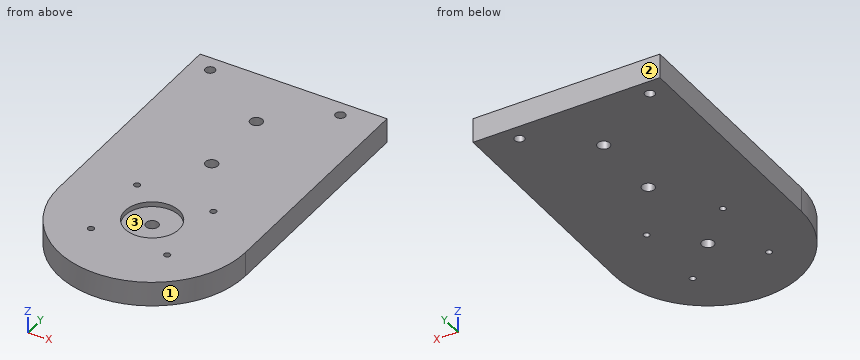
```python
from build123d import *

# Parameters (mm, degrees)
CROQUIS1_R              = 2.5
CROQUIS1_R_2            = 1.25
SALIENTE_EXTRUIR1_DEPTH = 10
CROQUIS3_R              = 11
CORTAR_EXTRUIR1_DEPTH   = 2
CROQUIS4_R              = 2
CORTAR_EXTRUIR2_DEPTH   = 103.805641869


with BuildPart() as part:
    # Croquis1 → Saliente-Extruir1 (new body)
    with BuildSketch(Plane.XY):
        with BuildLine():
            Line((-38, 0), (-38, 95))
            Line((-38, 95), (38, 95))
            Line((38, 95), (38, 0))
            ThreePointArc((38, 0), (0, -38), (-38, 0))
        make_face()
        with Locations((0, 40)):
            Circle(CROQUIS1_R, mode=Mode.SUBTRACT)
        Circle(CROQUIS1_R, mode=Mode.SUBTRACT)
        with Locations((0, 70)):
            Circle(CROQUIS1_R, mode=Mode.SUBTRACT)
        with Locations((-15.5, 15.5)):
            Circle(CROQUIS1_R_2, mode=Mode.SUBTRACT)
        with Locations((15.5, 15.5)):
            Circle(CROQUIS1_R_2, mode=Mode.SUBTRACT)
        with Locations((15.5, -15.5)):
            Circle(CROQUIS1_R_2, mode=Mode.SUBTRACT)
        with Locations((-15.5, -15.5)):
            Circle(CROQUIS1_R_2, mode=Mode.SUBTRACT)
    extrude(amount=SALIENTE_EXTRUIR1_DEPTH)

    # Croquis3 → Cortar-Extruir1 (cut)
    with BuildSketch(Plane.XY.offset(10)):
        Circle(CROQUIS3_R)
    extrude(amount=-CORTAR_EXTRUIR1_DEPTH, mode=Mode.SUBTRACT)

    # Croquis4 → Cortar-Extruir2 (cut, through all)
    with BuildSketch(Plane.XY.offset(10)):
        with Locations((-30, 88.5)):
            Circle(CROQUIS4_R)
        with Locations((23, 88.5)):
            Circle(CROQUIS4_R)
    extrude(amount=-CORTAR_EXTRUIR2_DEPTH, mode=Mode.SUBTRACT)


solid = part.part
```
Source: CAD feature listing. Evaluate the final solid. Frame: model axes, mm. Face numbers are marked on the shaded views. Coordinates: 2 decimals unless noted, no trailing zeros. Loops run counter-clockwise (first coordinate to the right, second up) from the corner with the lowest first, then second, coordinate; pieces in that order, holes last. Notation, with made-up numbers: M -25.75,77 L 20.25,77 A25 cw 20.25,96 Z; hole C 33.25,-14 d8. An arc over 180 degrees is marked long. Use a Markdown table: item, result. Add a question column.
Q1. Draft query along Y for the marked faces 1, 2 and 3. Return one class per face: pulls with the +Y half, pulls with the -Y half, needs draft (parallel to the pull), parting line crosses it, or undercut.
Q2. Section query C-C, the plane y = 40. Return loops of the section in (x, z), and give its area (3 significant figures).
Q3. Section query B-B, the plane x = -30. Return loops of the section in (y, z).
Q4. Material intervals for L1, parallel to Y at x = 0, z = 9.65; L2, parallel to Y at x = 0, z = 5.5; L3, parallel to Y at x = 15.5, z = 6, sorted ascending.
Q5. First-contact query: pin 1 (6.5 mm diameter, centred on x = -4, y = 5, fed in from +Z). Flat tip, straight axial feed; report the tip coordinate or a pass-through.
Q6. Section query D-D, the plane z = 6.5. State how many separate pieces and enclosed holes the cut face has, and give its area (3 significant figures).
Q7. Section query A-A, the plane y = 15.5. Return loops of the section in (x, z), and give its area (3 significant figures).
Result:
| question | item | result |
|---|---|---|
| 1 | face 1 | pulls with the -Y half |
| 1 | face 2 | pulls with the +Y half |
| 1 | face 3 | undercut |
| 2 | outline | M -38,0 L -2.5,0 L -2.5,10 L -38,10 Z; M 2.5,0 L 38,0 L 38,10 L 2.5,10 Z |
| 2 | area | 710 mm2 |
| 3 | outline | M -23.32,0 L 86.5,0 L 86.5,10 L -23.32,10 Z; M 90.5,0 L 95,0 L 95,10 L 90.5,10 Z |
| 4 | L1 | y = -38 to -11, 11 to 37.5, 42.5 to 67.5, 72.5 to 95 |
| 4 | L2 | y = -38 to -2.5, 2.5 to 37.5, 42.5 to 67.5, 72.5 to 95 |
| 4 | L3 | y = -34.7 to -16.75, -14.25 to 14.25, 16.75 to 95 |
| 5 | pin 1 | stops at z = 8 |
| 6 | separate pieces | 1 |
| 6 | enclosed holes | 9 |
| 6 | area | 9,380 mm2 |
| 7 | outline | M -38,0 L -16.75,0 L -16.75,10 L -38,10 Z; M -14.25,0 L 14.25,0 L 14.25,10 L -14.25,10 Z; M 16.75,0 L 38,0 L 38,10 L 16.75,10 Z |
| 7 | area | 710 mm2 |
